Answer from the drawing. Dimensions are ordinates in mm from the lowest x, y and z of the part. A direction names the side the tool comes from. Round coordinates to 2 decimals unless told otherwise and drop trailing zeros. Write each loop counter-clockwise with the first axis right and the second up, starting at its lowest first coordinate (ties: lowest second). Pieces come first, ordered by that corner, then holes.
1. Determine the mould class of the marked faces 1, 2 and 3 for opening direction X: pulls with the +X half, pulls with the -X half, needs draft (parallel to the pull), parting line crosses it, or undercut.
2. Flat-ended cylindrical pins translate along their axes: pin 1 Ø12 at (y, z) = (29, 65) entering from -X; pin 2 Ø12 at (x, z) = (32, 67) entering from -Y; pin 3 Ø10 at (x, z) = (57.183, 19.017) entering from +Y; pin 4 Ø14 at (y, z) = (51, 46) entering from +X. Find the tip coordinate at first contact, or state that the pin passes through.
3. A tool of negligible diameter and unlimited length cuts with its end or side. For the marked faces 4 and 5, from which of +Z, -Z, +X, -X, +Y, -Y can it reach the whole face along a straight path? Write none if from no direction.
4. Find section A-A (z = 38.1). Count the separate pieces of the cut face and the enclosed holes in it.
5. Straight lines are drawn through the part: probe 1 along X at (y, z) = (45, 37.5); probe 2 along Z at (x, y) = (38.1, 52.5); probe 3 along Z at (x, y) = (40.5, 52.5) (1 decimal). For each, find the intervals that lie inside material, in ascending order.
6. Find section D-D (x = 9). Write down the section's boundary in (y, z).
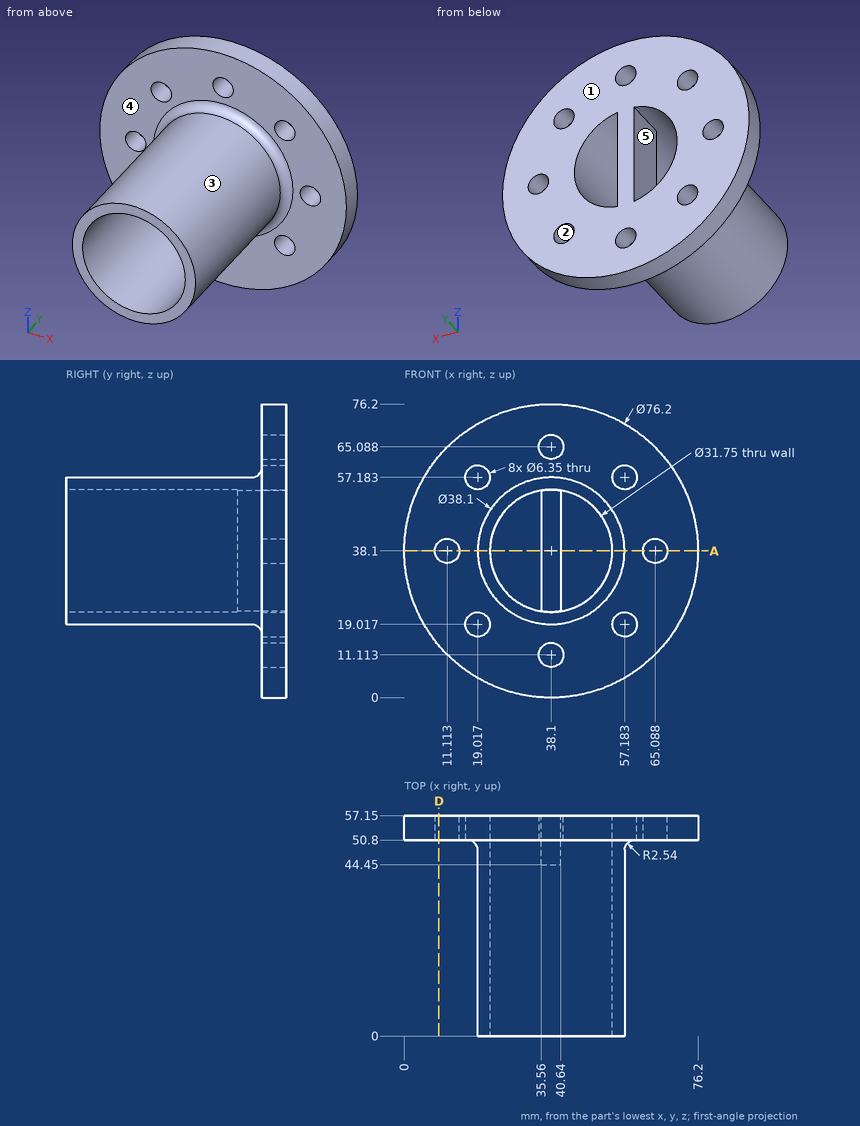
Worked answers:
1. face 1: needs draft
1. face 2: undercut
1. face 3: parting line crosses it
2. pin 1: passes through
2. pin 2: stops at y = 50.8
2. pin 3: stops at y = 57.15
2. pin 4: stops at x = 76.19
3. face 4: -Y
3. face 5: +Y, -Y
4. separate pieces: 5
4. enclosed holes: 0
5. probe 1: x = 19.06 to 22.24, 35.56 to 40.64, 53.96 to 57.14
5. probe 2: z = 0 to 7.94, 14.29 to 61.91, 68.26 to 76.2
5. probe 3: z = 0.1 to 9, 13.2 to 63, 67.2 to 76.1
6. outline: (50.8, 13.51) - (57.15, 13.51) - (57.15, 35.73) - (50.8, 35.73) - close; (50.8, 40.47) - (57.15, 40.47) - (57.15, 62.69) - (50.8, 62.69) - close
